Source: CAD feature listing. Evaluate the final solid. Frame: model axes, mm. A direction names the side the tool comes from. Give positions to 0.01 mm unless a question says otherwise; leave off trailing zeros. Order: outer loops, then holes, each group sorted by start corner. A loop starts at its lowest first (then second) coordinate and runs counter-clockwise, first axis right, second up. Notation, with made-up numbers: (19, 5) -> (39, 5) arc R22 ccw to (39, 13) -> close; hole circle Ø5 at (68, 60.5). An arc over 180 degrees is marked (long way). Use CSV: the item, a comma, the result in double quotes.
```python
from build123d import *

# Parameters (mm, degrees)
PAD_DEPTH    = 25
SKETCH001_W  = 30
SKETCH001_H  = 30
PAD001_DEPTH = 15


with BuildPart() as part:
    # Sketch → Pad (new body, symmetric)
    with BuildSketch(Plane.XZ):
        Polygon((-25, 25), (-25, -25), (25, -25), align=None)
    extrude(amount=PAD_DEPTH, both=True)

    # Sketch001 → Pad001 (join, symmetric)
    with BuildSketch(Plane.XZ):
        Rectangle(SKETCH001_W, SKETCH001_H)
    extrude(amount=PAD001_DEPTH, both=True)


solid = part.part
```
1. Ray query, line 1 along Z through (x, y) = (-3, 7); line 2 along Y through (x, z) = (8.5, 5.5). Return the intervals inside material, ascending.
Answer below:
line 1,"z = -25 to 15"
line 2,"y = -15 to 15"
2. Section query A-A on x = -8. Return loops of the section in (y, z), plus the area to 3 significant figures.
Answer below:
outline,"(-25, -25) -> (25, -25) -> (25, 8) -> (15, 8) -> (15, 15) -> (-15, 15) -> (-15, 8) -> (-25, 8) -> close"
area,"1,860 mm²"
3. Section query B-B on z = -7. Return loops of the section in (x, y).
Answer below:
outline,"(-25, -25) -> (7, -25) -> (7, -15) -> (15, -15) -> (15, 15) -> (7, 15) -> (7, 25) -> (-25, 25) -> close"
4. Section query C-C on y = 8. Return loops of the section in (x, z), plus the area to 3 significant figures.
Answer below:
outline,"(-25, -25) -> (25, -25) -> (15, -15) -> (15, 15) -> (-15, 15) -> (-25, 25) -> close"
area,"1,700 mm²"
5. Section query D-D on x = -22. Return loops of the section in (y, z), plus the area to 3 significant figures.
Answer below:
outline,"(-25, -25) -> (25, -25) -> (25, 22) -> (-25, 22) -> close"
area,"2,350 mm²"
6. Access query for faces 1 (the flat face through (6, -15, 7)), 2 (the flat face through (-11, -25, -11)), 3 (the flat face through (-11, 25, -11)), 4 (the flat face through (6, 15, 7)), 5 (the flat face through (15, 0, 0)). Directions: +Z, -Z, +X, -X, +Y, -Y. A direction counts if a zero-diameter tool reaches every point of the face in a straight line with its end or side. Return the directions, or none.
Answer below:
face 1,"+Z, +X, -Y"
face 2,"+Z, -Z, +X, -X, -Y"
face 3,"+Z, -Z, +X, -X, +Y"
face 4,"+Z, +X, +Y"
face 5,"+Z, +X, +Y, -Y"
7. Pin query (flat end, axial travel): P1, Ø8, axis at y = 0, z = 2, coming from the +X side; P2, Ø10, axis at x = -16.5, y = -12.5, coming from the +Z side; P3, Ø12, axis at x = 14, z = -1, coming from the +Y side. Return the tip coordinate at first contact, or that it passes through.
Answer below:
P1,"stops at x = 15"
P2,"stops at z = 21.5"
P3,"stops at y = 15"
